Part model, mm, in its own coordinate system. A direction names the side the tool comes from. Give positions to 0.01 mm unless a question says otherwise; leave off trailing zeros. Write each loop counter-clockwise with the first axis right and the second up, starting at its lowest first coordinate (ties: lowest second). Pieces come first, ordered by that corner, then holes.
from build123d import *

# Parameters (mm, degrees)
F1_DEPTH = 80
F2_SIZE  = 30
F3_T     = -1.6
F4_W     = 95
F4_H     = 118.4
F4_H_2   = 60
F5_DEPTH = 25
F6_W     = 80
F6_H     = 100
F7_DEPTH = 25


with BuildPart() as f1:
    # F0 (on Front) → F1 (new body, symmetric)
    with BuildSketch(Plane.XZ):
        Polygon((50, -90), (90, -90), (90, 90), (-90, 90), (-90, -90), (-50, -90), (-50, 60), (0, 60), (50, 60), align=None)
    extrude(amount=F1_DEPTH, both=True)

    # F2
    f2_edges = [f1.edges().sort_by_distance(p)[0] for p in [
        (-90, -80, 0),
        (90, -80, 0),
        (90, 80, 0),
        (-90, 80, 0),
    ]]
    chamfer(f2_edges, length=F2_SIZE)

    # F3
    f3_openings = [f1.faces().sort_by_distance(p)[0] for p in [
        (68.363636, 0, -90),
        (-68.363636, 0, -90),
        (0, 0, 60),
        (50, 0, -15),
        (-50, 0, -15),
    ]]
    offset(amount=F3_T, openings=f3_openings)

    # F4 (on face) → F5 (cut)
    with BuildSketch(Plane.YZ.offset(90)):
        with Locations((0, -30.8)):
            Rectangle(F4_W, F4_H)
        with Locations((0, 58.4)):
            Rectangle(F4_W, F4_H_2)
    extrude(amount=-F5_DEPTH, mode=Mode.SUBTRACT)

    # F6 (on face) → F7 (cut)
    with BuildSketch(Plane.XY.offset(90)):
        Rectangle(F6_W, F6_H)
    extrude(amount=-F7_DEPTH, mode=Mode.SUBTRACT)


solid = f1.part
1) Flat gauge pins, fed straight in: P1, Ø8, axis at y = 62.5, z = -24.5, coming from the +X side; P2, Ø1.8, axis at y = -79.5, z = -51.5, coming from the +X side; P3, Ø0.8, axis at x = -8, y = 79, coming from the -Z side. Where does each tip first touch, or does it go through?
Check result:
P1: stops at x = 81.5
P2: stops at x = 61.4
P3: stops at z = 60
2) Mould opens along Y. For faces 1 (the flat face through (41, -1, 90)), 2 (the flat face through (0, 78.4, 66)), 3 (the flat face through (-75, 65, 1)) say: +Y half, -Y half, draft (parallel to the pull), parting line (faces both ways), or undercut.
Check result:
face 1: draft
face 2: undercut
face 3: +Y half
3) Saw through at A-A (x = 18). Write the cut outline in (y, z).
Check result:
outline: (-80, 60) - (-78.4, 60) - (-78.4, 88.4) - (-50, 88.4) - (-50, 90) - (-80, 90) - close; (50, 88.4) - (78.4, 88.4) - (78.4, 60) - (80, 60) - (80, 90) - (50, 90) - close
4) Saw through at C-C (z = -73.5). Write the cut outline in (x, y).
Check result:
outline: (-90, -50) - (-60, -80) - (-50, -80) - (-50, -78.4) - (-59.34, -78.4) - (-88.4, -49.34) - (-88.4, 49.34) - (-59.34, 78.4) - (-50, 78.4) - (-50, 80) - (-60, 80) - (-90, 50) - close; (50, -80) - (60, -80) - (90, -50) - (90, -47.5) - (88.4, -47.5) - (88.4, -49.34) - (59.34, -78.4) - (50, -78.4) - close; (50, 78.4) - (59.34, 78.4) - (88.4, 49.34) - (88.4, 47.5) - (90, 47.5) - (90, 50) - (60, 80) - (50, 80) - close
5) Saw through at B-B (y = 37). Write the cut outline in (x, z).
Check result:
outline: (-90, -90) - (-88.4, -90) - (-88.4, 88.4) - (-40, 88.4) - (-40, 90) - (-90, 90) - close; (40, 88.4) - (90, 88.4) - (90, 90) - (40, 90) - close
6) Saw through at D-D (x = -46.5). Write the cut outline in (y, z), and give its area (3 significant figures).
Check result:
outline: (-80, 60) - (-78.4, 60) - (-78.4, 88.4) - (78.4, 88.4) - (78.4, 60) - (80, 60) - (80, 90) - (-80, 90) - close
area: 347 mm2
7) 3-axis set-ups, long thin cutter, end or side, ignore diameter. For faces 4 (the flat face through (-73.67, 64.07, 0.45)), 5 (the flat face through (75, 65, -1)): which of +Z, -Z, +X, -X, +Y, -Y reach the whole face in a straight line?
Check result:
face 4: -Z
face 5: +Z, -Z, +X, +Y
8) Drill centre lines: L1, parallel to Y at x = -51, z = -71; L2, parallel to X at y = -19, z = -17.5; L3, parallel to Z at x = -54.5, y = 9. Where is each one in solid material? Low to high.
Check result:
L1: y = -80 to -78.4, 78.4 to 80
L2: x = -90 to -88.4
L3: z = 88.4 to 90
